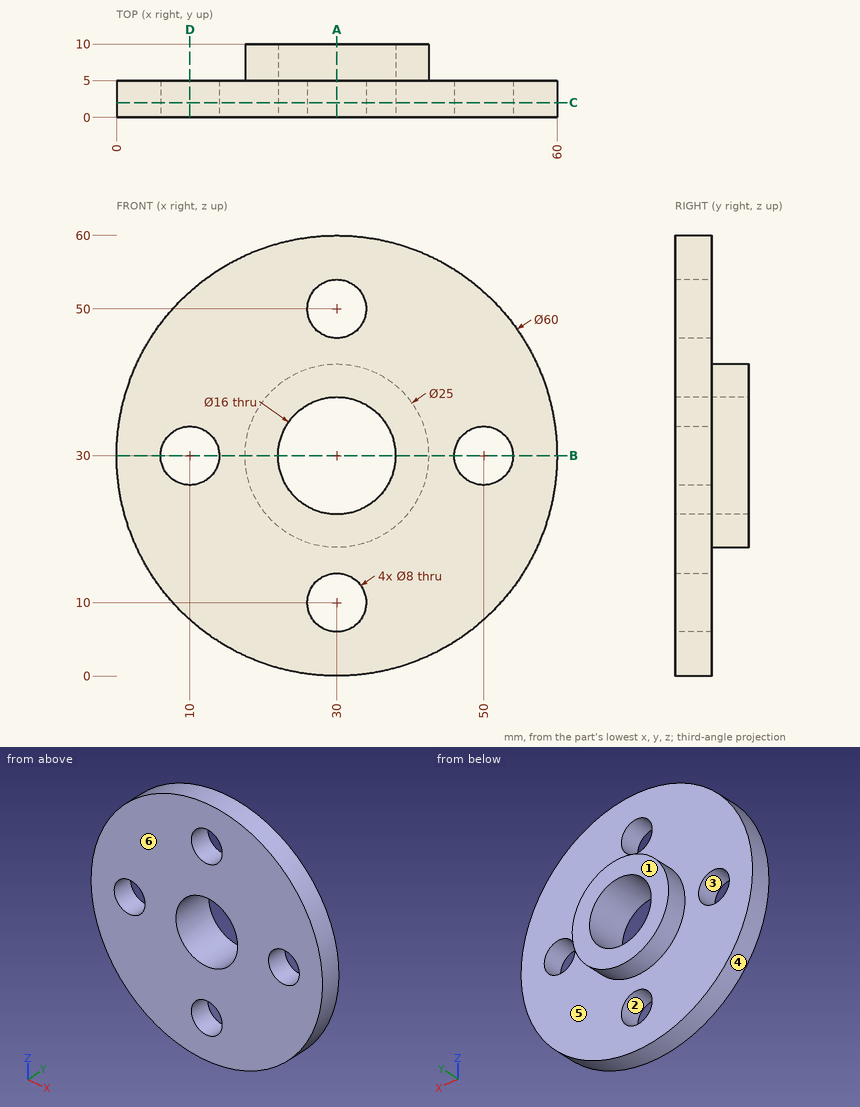
Print and shaded views of the part. All mm, measured from the part's lowest x, y and z. A direction names the side the tool comes from. Give positions to 0.01 mm unless a question says otherwise; leave off trailing zeros. Write each loop counter-clockwise with the first axis right and the second up, starting at its lowest first coordinate (ties: lowest second). Pieces come first, ordered by that corner, then holes. Notation, with made-up numbers: (-33.5, 85.25) -> (-19.5, 85.25) arc R23 cw to (-19.5, 123.25) -> close; hole circle Ø2 at (40.5, 85.25). An arc over 180 degrees is marked (long way). Use CSV: the item, a comma, the result in double quotes. Start each with the question number.
1) Cut at D-D on x = 10. List the corners of the cut face in (y, z), plus the area to 3 significant figures.
2) Cut at C-C on y = 2. List the corners of the cut face in (x, z).
3) Tool access for the marked faces 5 and 6: list every direction of +Z, -Z, +X, -X, +Y, -Y with a clear straight run to the whole face (end or side of a thin tool).
4) Cut at A-A on x = 30. List the corners of the cut face in (y, z), plus the area to 3 significant figures.
5) Cut at B-B on z = 30. List the corners of the cut face in (x, y).
6) Pin check, flat tips, straight feed: P1, Ø6, axis at y = 2, z = 21.5, coming from the -X side; P2, Ø1.5, axis at x = 28.5, y = 7, coming from the -Z side; P3, Ø1.5, axis at x = 49, y = 6, coming from the +Z side; P4, Ø1, axis at y = 4, z = 34, coming from the -X side. Stop position of each tip, or through.
7) Two-plate mould, pull along Z, no slides. Class the marked faces 1, 2, 3 and 4: released by +Z, released by -Z, zero draft, split by the parting line, or undercut.
8) Drill centre lines: L1, parallel to X at y = 6.75, z = 30; L2, parallel to Y at x = 20.5, z = 13; L3, parallel to X at y = 1.4, z = 10. Where is each one in solid material? Low to high.
Final values:
1,outline,"(0, 7.64) -> (5, 7.64) -> (5, 26) -> (0, 26) -> close; (0, 34) -> (5, 34) -> (5, 52.36) -> (0, 52.36) -> close"
1,area,"184 mm2"
2,outline,"circle Ø60 at (30, 30); hole circle Ø8 at (10, 30); hole circle Ø16 at (30, 30); hole circle Ø8 at (30, 10); hole circle Ø8 at (30, 50); hole circle Ø8 at (50, 30)"
3,face 5,"+Y"
3,face 6,"+Z, -Z, +X, -X, -Y"
4,outline,"(0, 0) -> (5, 0) -> (5, 6) -> (0, 6) -> close; (0, 14) -> (5, 14) -> (5, 17.5) -> (10, 17.5) -> (10, 22) -> (0, 22) -> close; (0, 38) -> (10, 38) -> (10, 42.5) -> (5, 42.5) -> (5, 46) -> (0, 46) -> close; (0, 54) -> (5, 54) -> (5, 60) -> (0, 60) -> close"
4,area,"185 mm2"
5,outline,"(0, 0) -> (6, 0) -> (6, 5) -> (0, 5) -> close; (14, 0) -> (22, 0) -> (22, 10) -> (17.5, 10) -> (17.5, 5) -> (14, 5) -> close; (38, 0) -> (46, 0) -> (46, 5) -> (42.5, 5) -> (42.5, 10) -> (38, 10) -> close; (54, 0) -> (60, 0) -> (60, 5) -> (54, 5) -> close"
6,P1,"stops at x = 0.51"
6,P2,"stops at z = 17.52"
6,P3,"passes through"
6,P4,"stops at x = 0.2"
7,face 1,"zero draft"
7,face 2,"undercut"
7,face 3,"undercut"
7,face 4,"split by the parting line"
8,L1,"x = 17.5 to 22, 38 to 42.5"
8,L2,"y = 0 to 5"
8,L3,"x = 7.64 to 26, 34 to 52.36"
